```python
from build123d import *

# Parameters (mm, degrees)
M14X1_5_TAPPED_HOLE1_D              = 12.5
M14X1_5_TAPPED_HOLE1_DEPTH          = 25.4
M14X1_5_TAPPED_HOLE1_TIP            = 3.755378869
F_1_16_0_0625_DIAMETER_HOLE1_D      = 1.5875
F_1_16_0_0625_DIAMETER_HOLE1_DEPTH  = 28.575
F_1_16_0_0625_DIAMETER_HOLE1_TIP    = 0.476933116
F_3_32_0_09375_DIAMETER_HOLE1_D     = 2.38125
F_3_32_0_09375_DIAMETER_HOLE1_DEPTH = 28.702
F_3_32_0_09375_DIAMETER_HOLE1_TIP   = 0.715399675
F_1_4_0_25_DIAMETER_HOLE1_D         = 6.35
CIRPATTERN1_COUNT                   = 6
F_1_32_0_03125_DIAMETER_HOLE1_D     = 0.79375
F_1_32_0_03125_DIAMETER_HOLE1_DEPTH = 28.575
F_1_32_0_03125_DIAMETER_HOLE1_TIP   = 0.238466558


with BuildPart() as part:
    # Sketch1 → Revolve1 (revolve)
    with BuildSketch(Plane.XY):
        Polygon((-3.81, 0), (-8.0645, 0), (-8.0645, 2.032), (-11.1125, 2.032), (-11.1125, 0), (-12.7, 0), (-12.7, -6.35), (-31.75, -6.35), (-31.75, 31.75), (-3.81, 31.75), align=None)
    revolve(axis=Axis((0, 0, 0), (0, 1, 0)))

    # M14x1.5 Tapped Hole1
    with Locations(Plane(origin=(0, 31.75, 0), x_dir=(1, 0, 0), z_dir=(0, 1, 0))):
        with Locations((0, 0)):
            Hole(M14X1_5_TAPPED_HOLE1_D / 2, depth=M14X1_5_TAPPED_HOLE1_DEPTH)
            with Locations((0, 0, -(M14X1_5_TAPPED_HOLE1_DEPTH + M14X1_5_TAPPED_HOLE1_TIP / 2))):  # 118° drill point
                Cone(0, M14X1_5_TAPPED_HOLE1_D / 2, M14X1_5_TAPPED_HOLE1_TIP, mode=Mode.SUBTRACT)

    # Sketch6 → 1/4 NPT Tapped Hole1 (revolve, cut)
    with BuildSketch(Plane(origin=(31.75, 12.7, 0), x_dir=(0, 0, -1), z_dir=(0, 1, 0))):
        Polygon((0, 0), (0, 20.360347279), (5.5626, 17.018), (5.5626, 9.906), (5.943685794, 9.906), (6.2402847, 0), align=None)
    revolve(axis=Axis((38.1, 12.7, 0), (-1, 0, 0)), mode=Mode.SUBTRACT)

    # Sketch8 → 1/4 NPT Tapped Hole2 (revolve, cut)
    with BuildSketch(Plane(origin=(-31.75, 12.7, 0), x_dir=(0, 0, 1), z_dir=(0, 1, 0))):
        Polygon((0, 0), (0, 20.360347279), (5.5626, 17.018), (5.5626, 9.906), (5.943685794, 9.906), (6.2402847, 0), align=None)
    revolve(axis=Axis((-38.1, 12.7, 0), (1, 0, 0)), mode=Mode.SUBTRACT)

    # 1/16 (0.0625) Diameter Hole1
    with Locations(Plane(origin=(31.75, 0, 0), x_dir=(0, 0, -1), z_dir=(1, 0, 0))):
        with Locations((0, 12.7)):
            Hole(F_1_16_0_0625_DIAMETER_HOLE1_D / 2, depth=F_1_16_0_0625_DIAMETER_HOLE1_DEPTH)
            with Locations((0, 0, -(F_1_16_0_0625_DIAMETER_HOLE1_DEPTH + F_1_16_0_0625_DIAMETER_HOLE1_TIP / 2))):  # 118° drill point
                Cone(0, F_1_16_0_0625_DIAMETER_HOLE1_D / 2, F_1_16_0_0625_DIAMETER_HOLE1_TIP, mode=Mode.SUBTRACT)

    # 3/32 (0.09375) Diameter Hole1
    with Locations(Plane.ZY.offset(31.75)):
        with Locations((0, 12.7)):
            Hole(F_3_32_0_09375_DIAMETER_HOLE1_D / 2, depth=F_3_32_0_09375_DIAMETER_HOLE1_DEPTH)
            with Locations((0, 0, -(F_3_32_0_09375_DIAMETER_HOLE1_DEPTH + F_3_32_0_09375_DIAMETER_HOLE1_TIP / 2))):  # 118° drill point
                Cone(0, F_3_32_0_09375_DIAMETER_HOLE1_D / 2, F_3_32_0_09375_DIAMETER_HOLE1_TIP, mode=Mode.SUBTRACT)

    # 1/4 (0.25) Diameter Hole1 (through all)
    with Locations(Plane(origin=(0, 31.75, 0), x_dir=(1, 0, 0), z_dir=(0, 1, 0))):
        with Locations((21.997045256, 12.7)):
            f_1_4_0_25_diameter_hole1 = Hole(F_1_4_0_25_DIAMETER_HOLE1_D / 2)

    # CirPattern1: 1/4 (0.25) Diameter Hole1 ×6 about axis
    cirpattern1_axis = Axis((0, 0, 0), (0, 1, 0))
    for i in range(1, CIRPATTERN1_COUNT):
        add(f_1_4_0_25_diameter_hole1.rotate(cirpattern1_axis, i * 360 / CIRPATTERN1_COUNT), mode=Mode.SUBTRACT)

    # Sketch18 → 1/4 NPT Tapped Hole3 (revolve, cut)
    with BuildSketch(Plane(origin=(15.875, 12.7, -27.49630657), x_dir=(-0.866025404, 0, -0.5), z_dir=(0, 1, 0))):
        Polygon((0, 0), (0, 19.852347279), (5.5626, 16.51), (5.5626, 12.7), (6.557983593, 12.7), (6.9382386, 0), align=None)
    revolve(axis=Axis((19.05, 12.7, -32.995567884), (-0.5, 0, 0.866025404)), mode=Mode.SUBTRACT)

    # 1/32 (0.03125) Diameter Hole1
    with Locations(Plane(origin=(15.875, 0, -27.49630657), x_dir=(0, -1, 0), z_dir=(0.5, 0, -0.866025404))):
        with Locations((-12.7, 0)):
            Hole(F_1_32_0_03125_DIAMETER_HOLE1_D / 2, depth=F_1_32_0_03125_DIAMETER_HOLE1_DEPTH)
            with Locations((0, 0, -(F_1_32_0_03125_DIAMETER_HOLE1_DEPTH + F_1_32_0_03125_DIAMETER_HOLE1_TIP / 2))):  # 118° drill point
                Cone(0, F_1_32_0_03125_DIAMETER_HOLE1_D / 2, F_1_32_0_03125_DIAMETER_HOLE1_TIP, mode=Mode.SUBTRACT)


solid = part.part
```
Read the model definition and answer for the solid it produces. Units are mm, in the model's axes. A direction names the side the tool comes from. Give positions to 0.01 mm unless a question says otherwise; leave off trailing zeros. Write each loop counter-clockwise with the first axis right and the second up, starting at its lowest first coordinate (ties: lowest second). Pieces come first, ordered by that corner, then holes. Notation, with made-up numbers: (-26, 21.5) -> (-19, 21.5) arc R9 cw to (-19, 36.5) -> close; hole circle Ø11 at (59.25, 60.5). An arc over 180 degrees is marked (long way). Answer in a Markdown table with one row per item.
1) Section A-A on z = 25.4 is taken. Give the vertices of the cut face in (x, y) (3 decimals), plus the area to 3 significant figures.
Results list:
| item | result |
|---|---|
| outline | (-19.05, -6.35) -> (-3.175, -6.35) -> (-3.175, 31.75) -> (-19.05, 31.75) -> close; (3.175, -6.35) -> (19.05, -6.35) -> (19.05, 31.75) -> (3.175, 31.75) -> close |
| area | 1,210 mm^2 |
2) A tool of negligible diameter and unlimited length cuts with its end or side. For faces 1 (the flat face through (-1.9, 0, -3.5)), 2 (the cylindrical face through (18.338, 7.185, 0.724)), 3 (the cylindrical face through (4.8, 12.4, -7.8)), 4 (the flat face through (-21.844, 14.9, -5.3)), from which of +Z, -Z, +X, -X, +Y, -Y can it reach the whole face along a straight path? Write none if from no direction.
Results list:
| item | result |
|---|---|
| face 1 | -Y |
| face 2 | +X |
| face 3 | none |
| face 4 | -X |
3) Section B-B on x = 0 is taken. Count the separate pieces of the cut face and the enclosed holes in it, plus the area to 3 significant figures.
Results list:
| item | result |
|---|---|
| separate pieces | 4 |
| enclosed holes | 0 |
| area | 1,390 mm^2 |
4) Straight lines are drawn through the part: line 1 (Z direction, x = 0, y = 3) (3 decimals); line 2 (Z direction, x = 0, y = 30) (3 decimals); line 3 (X direction, y = 16, z = -12). For each, find the intervals that lie inside material, in ascending order. Write a range as [from, to].
Results list:
| item | result |
|---|---|
| line 1 | [-31.75, -28.575], [-22.225, -3.81], [3.81, 22.225], [28.575, 31.75] |
| line 2 | [-31.75, -28.575], [-22.225, -6.25], [6.25, 22.225], [28.575, 31.75] |
| line 3 | [-29.39, -25.09], [-18.9, 6.98], [12.1, 18.9], [25.09, 29.39] |
5) Determine the mould class of faces 5 (the cylindrical face through (-18.338, 7.185, -0.724)), 6 (the flat face through (-7, 31.75, 0)) for opening direction Z: released by +Z, released by -Z, zero draft, split by the parting line, or undercut.
Results list:
| item | result |
|---|---|
| face 5 | undercut |
| face 6 | zero draft |
6) Each of these flat-tipped pins is pushed along its axis until it touches: pin 1 Ø2 at (y, z) = (9.5, 11.5) entering from +X; pin 2 Ø17.5 at (x, z) = (-0.5, -3.5) entering from -Y; pin 3 Ø7.5 at (x, z) = (-22, -12.7) entering from +Y; pin 4 Ø5 at (x, z) = (-22, 12.7) entering from +Y. Where does it stop, or does it pass through?
Results list:
| item | result |
|---|---|
| pin 1 | x = 29.96 |
| pin 2 | y = 0 |
| pin 3 | y = 31.75 |
| pin 4 | through |
